Source: CAD feature listing. Evaluate the final solid. Frame: model axes, mm. A direction names the side the tool comes from. Round coordinates to 2 decimals unless told otherwise and drop trailing zeros. Order: outer loops, then holes, each group sorted by start corner. A loop starts at its lowest first (then second) coordinate and runs counter-clockwise, first axis right, second up. Notation, with made-up numbers: (-10, 49) - (27, 49) arc R12 ccw to (27, 59) - close; hole circle Ø7 at (38.25, 12.25). An arc over 180 degrees is marked (long way). Use one line per item in the form item = value. Start each with the question number.
Q1. Cut plane B-B, the plane y = -0.5. Return the cut outline in (x, z), and give its area (3 significant figures).
Q2. Ray query, line 1 (X direction, y = -4.5, z = 0.6); line 2 (X direction, y = 2.75, z = 1.05); line 3 (Z direction, x = -0.95, y = -8.25). Return the intervals inside material, ascending. Write a range as [from, to].
Q3. Set-up query: faces 1 (the cylindrical face through (-0.08, -5.02, -1.813)), 2 (the cylindrical face through (-1.48, 1.23, -1.94)), 3 (the cylindrical face through (0.08, 7.407, -1.813)). Return all of +Z, -Z, +X, -X, +Y, -Y with unobstructed straight access to the full face (end or side cutting, diameter ignored); none if empty.
Q4. Cut plane A-A, the plane y = 6. Return the cut outline in (x, z) (3 decimals), and give its area (3 significant figures).
from build123d import *

# Parameters (mm, degrees)
CROQUIS1_R              = 2.44
SALIENTE_EXTRUIR1_DEPTH = 2.5
CROQUIS2_R              = 1.815
SALIENTE_EXTRUIR2_DEPTH = 10
SALIENTE_EXTRUIR3_START = 10
CROQUIS3_R              = 1.815
SALIENTE_EXTRUIR3_DEPTH = 10
REDONDEO1_R             = 1
REDONDEO2_R             = 1


with BuildPart() as part:
    # Croquis1 → Saliente-Extruir1 (new body)
    with BuildSketch(Plane(origin=(0, 0, 0), x_dir=(1, 0, 0), z_dir=(0, 1, 0))):
        with Locations(Location((0, 0, 0), (0, 0, 270))):
            Circle(CROQUIS1_R)
    extrude(amount=SALIENTE_EXTRUIR1_DEPTH)

    # Croquis2 → Saliente-Extruir2 (add)
    with BuildSketch(Plane(origin=(0, 2.5, 0), x_dir=(1, 0, 0), z_dir=(0, 1, 0))):
        with Locations(Location((0, 0, 0), (0, 0, 270))):
            Circle(CROQUIS2_R)
    extrude(amount=SALIENTE_EXTRUIR2_DEPTH)

    # Croquis3 → Saliente-Extruir3 (add)
    with BuildSketch(Plane.XZ.offset(SALIENTE_EXTRUIR3_START)):
        with Locations(Location((0, 0, 0), (0, 0, 90))):
            Circle(CROQUIS3_R)
    extrude(amount=-SALIENTE_EXTRUIR3_DEPTH)

    # Redondeo1
    # the kernel refuses this fillet: 1 mm, written as the material it adds along each edge
    with BuildSketch(Plane(origin=(0, 0, 0), x_dir=(0, 0, 1), z_dir=(1, 0, 0))) as redondeo1_piece_1:
        with BuildLine():
            CenterArc((2.815, 0.927024811), REDONDEO1_R, 180, 67.975687163)
            Line((1.815, 0.927024811), (1.795, 0.927024811))
            Line((1.795, 0.927024811), (1.795, 0))
            Line((1.795, 0), (1.815, -0.02))
            ThreePointArc((1.815, -0.02), (2.1275, -0.02), (2.4325, -0.018540496))
            Line((2.4325, -0.018540496), (2.44, 0))
        make_face()
    revolve(axis=Axis((0, 0, 0), (0, -1, 0)))
    with BuildSketch(Plane(origin=(0, 2.5, 0), x_dir=(0, 0, 1), z_dir=(-1, 0, 0))) as redondeo1_piece_2:
        with BuildLine():
            CenterArc((2.815, 0.927024811), REDONDEO1_R, 180, 67.975687163)
            Line((1.815, 0.927024811), (1.795, 0.927024811))
            Line((1.795, 0.927024811), (1.795, 0))
            Line((1.795, 0), (1.815, -0.02))
            ThreePointArc((1.815, -0.02), (2.1275, -0.02), (2.4325, -0.018540496))
            Line((2.4325, -0.018540496), (2.44, 0))
        make_face()
    revolve(axis=Axis((0, 2.5, 0), (0, 1, 0)))

    # Redondeo2
    redondeo2_edges = [part.edges().sort_by_distance(p)[0] for p in [
        (0, -10, -1.815),
        (0, 12.5, -1.815),
    ]]
    fillet(redondeo2_edges, radius=REDONDEO2_R)


solid = part.part
Completed:
q1.outline = circle Ø3.82 at (0, 0)
q1.area = 11.5 mm2
q2.line_1 = [-1.71, 1.71]
q2.line_2 = [-1.79, 1.79]
q2.line_3 = [-1.55, 1.55]
q3.face_1 = -Y
q3.face_2 = +Y, -Y
q3.face_3 = +Y
q4.outline = circle Ø3.63 at (0, 0)
q4.area = 10.3 mm2
